Here's how the part is built. I have some questions about the finished solid (model axes, mm). Face numbers are marked on the shaded views. A direction names the side the tool comes from. Give positions to 0.01 mm unless a question says otherwise; leave off trailing zeros. Loops run counter-clockwise (first coordinate to the right, second up) from the corner with the lowest first, then second, coordinate; pieces in that order, holes last. Notation, with made-up numbers: (37, 59.25) - (52, 59.25) arc R19 cw to (52, 91.25) - close; hole circle Ø8 at (-3, 69). An arc over 180 degrees is marked (long way). One line per item, written item: value. Start each with the question number.
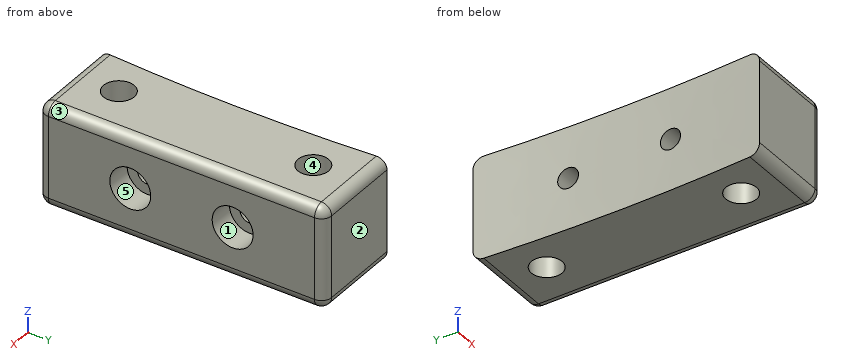
```python
from build123d import *

# Parameters (mm, degrees)
CYLINDER001_R     = 4
CYLINDER001_DEPTH = 5
CYLINDER_R        = 4
CYLINDER_DEPTH    = 5
SKETCH002_R       = 2
PAD002_DEPTH      = 18
SKETCH001_R       = 2
PAD001_DEPTH      = 18
SKETCH_R          = 3
PAD_DEPTH         = 20
FILLET_R          = 2


with BuildPart() as cylinder001:
    # Cylinder001 → Cylinder001 (new body)
    with BuildSketch(Plane(origin=(18, 38, 10), x_dir=(0, 0, 1), z_dir=(-1, 0, 0))):
        Circle(CYLINDER001_R)
    extrude(amount=CYLINDER001_DEPTH)


with BuildPart() as cylinder:
    # Cylinder → Cylinder (new body)
    with BuildSketch(Plane(origin=(18, 18, 10), x_dir=(0, 0, 1), z_dir=(-1, 0, 0))):
        Circle(CYLINDER_R)
    extrude(amount=CYLINDER_DEPTH)


with BuildPart() as body002:
    # Sketch002 → Pad002 (new body)
    with BuildSketch(Plane.YZ):
        with Locations((18, 10)):
            Circle(SKETCH002_R)
    extrude(amount=PAD002_DEPTH)


with BuildPart() as body002_1:
    # Body002 placement: moved
    add(body002.part.moved(Location((0, 20, 0))))


with BuildPart() as body001:
    # Sketch001 → Pad001 (new body)
    with BuildSketch(Plane.YZ):
        with Locations((18, 10)):
            Circle(SKETCH001_R)
    extrude(amount=PAD001_DEPTH)


with BuildPart() as fillet_body:
    # Sketch → Pad (new body)
    with BuildSketch(Plane.XY):
        with BuildLine():
            Line((0, 0), (18, 0))
            Line((18, 0), (18, 56))
            Line((18, 56), (0, 56))
            add(Edge.make_bspline(
                [(0, 0), (2, 28), (0, 56)],
                knots=[0, 0, 0, 1, 1, 1], degree=2))
        make_face()
        with Locations((8, 47)):
            Circle(SKETCH_R, mode=Mode.SUBTRACT)
        with Locations((8, 9)):
            Circle(SKETCH_R, mode=Mode.SUBTRACT)
    extrude(amount=PAD_DEPTH)

    # Boolean: cut Body002, Body001
    add(body002_1.part, mode=Mode.SUBTRACT)
    add(body001.part, mode=Mode.SUBTRACT)

    # Cut: cut Cylinder
    add(cylinder.part, mode=Mode.SUBTRACT)

    # Cut001: cut Cylinder001
    add(cylinder001.part, mode=Mode.SUBTRACT)

    # Fillet
    fillet_edges = [fillet_body.edges().sort_by_distance(p)[0] for p in [
        (18, 0, 10),
        (9, 0, 0),
        (9, 0, 20),
        (18, 28, 0),
        (18, 28, 20),
        (18, 56, 10),
        (9, 56, 0),
        (9, 56, 20),
    ]]
    fillet(fillet_edges, radius=FILLET_R)


solid = fillet_body.part
```
(1) If we section it at C-C on z = 10: Give the number of separate pieces and of enclosed holes in the cut face, plus the area to 3 significant figures.
(2) If we mould it in two halves opening along X, with no side actions, what happens to the marked faces 3, 4 and 5? For each: pulls with the +X half, pulls with the -X half, needs draft (parallel to the pull), parting line crosses it, or undercut.
(3) If we section it at A-A on x = 8: List the corners of the cut face in (y, z) for me.
(4) If we section it at B-B on x = 15.5: List the corners of the cut face in (y, z) for me, plus the area to 3 significant figures.
(5) For the marked faces 1 and 2, which set-ups out of +Z, -Z, +X, -X, +Y, -Y let a thin tool reach every point of the face, with its end or its side?
(6) Will these pins go through, and if not, where does the flat tip stop? pin 1 (5.5 mm diameter, centred on x = 8, y = 47, fed in from -Z); pin 2 (7 mm diameter, centred on y = 38, z = 10, fed in from -X); pin 3 (2.5 mm diameter, centred on y = 36, z = 9, fed in from +X); pin 4 (8 mm diameter, centred on y = 44.5, z = 8.5, fed in from -X).
(7) Please list where these lines run through material, in increasing order: probe 1 along Y at (x, z) = (8.25, 4.75); probe 2 along Y at (x, z) = (13.75, 10); probe 3 along Y at (x, z) = (8, 9.25). Write a range as from..to.
Found:
1. separate pieces: 3
1. enclosed holes: 2
1. area: 735 mm^2
2. face 3: pulls with the +X half
2. face 4: undercut
2. face 5: needs draft
3. outline: (0, 2) arc R2 ccw to (2, 0) - (6, 0) - (6, 20) - (2, 20) arc R2 ccw to (0, 18) - close; (12, 0) - (44, 0) - (44, 20) - (12, 20) - close; (50, 0) - (54, 0) arc R2 ccw to (56, 2) - (56, 18) arc R2 ccw to (54, 20) - (50, 20) - close; hole circle Ø4 at (18, 10); hole circle Ø4 at (38, 10)
4. outline: (0, 2) arc R2 ccw to (2, 0) - (54, 0) arc R2 ccw to (56, 2) - (56, 18) arc R2 ccw to (54, 20) - (2, 20) arc R2 ccw to (0, 18) - close; hole circle Ø8 at (18, 10); hole circle Ø8 at (38, 10)
4. area: 1,020 mm^2
5. face 1: +X
5. face 2: +Z, -Z, +X, -X, +Y
6. pin 1: through
6. pin 2: x = 0.77
6. pin 3: x = 13
6. pin 4: x = 0.46
7. probe 1: 0..6.01, 11.99..44.01, 49.99..56
7. probe 2: 0..14, 22..34, 42..56
7. probe 3: 0..6, 12..16.15, 19.85..36.15, 39.85..44, 50..56
